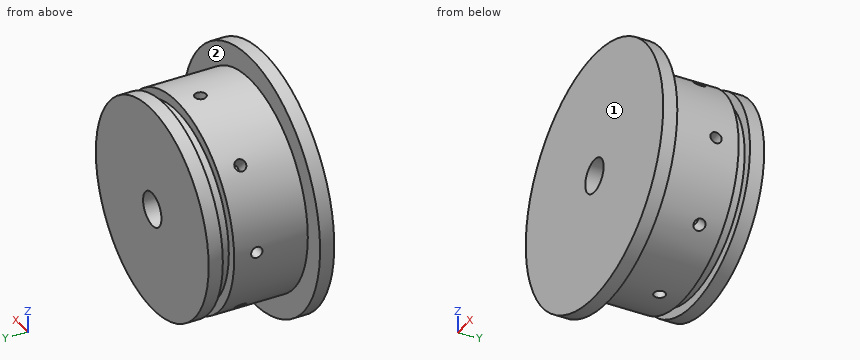
```python
from build123d import *

# Parameters (mm, degrees)
SKETCH1_R           = 45
BOSS_EXTRUDE1_DEPTH = 40
SKETCH2_R           = 45
SKETCH2_R_2         = 36.95
CUT_EXTRUDE1_DEPTH  = 35
SKETCH5_W           = 3.5
SKETCH5_H           = 4
SKETCH6_R           = 2
CUT_EXTRUDE4_DEPTH  = 46
SKETCH8_R           = 2
BOSS_EXTRUDE2_DEPTH = 30
CIRPATTERN1_COUNT   = 8
SKETCH4_R           = 6
CUT_EXTRUDE3_DEPTH  = 77


with BuildPart() as part:
    # Sketch1 → Boss-Extrude1 (new body)
    with BuildSketch(Plane(origin=(0, 0, 0), x_dir=(1, 0, 0), z_dir=(0, 1, 0))):
        Circle(SKETCH1_R)
    extrude(amount=BOSS_EXTRUDE1_DEPTH)

    # Sketch2 → Cut-Extrude1 (cut)
    with BuildSketch(Plane(origin=(0, 40, 0), x_dir=(1, 0, 0), z_dir=(0, 1, 0))):
        Circle(SKETCH2_R)
        Circle(SKETCH2_R_2, mode=Mode.SUBTRACT)
    extrude(amount=-CUT_EXTRUDE1_DEPTH, mode=Mode.SUBTRACT)

    # Sketch5 → Cut-Revolve1 (revolve, cut)
    with BuildSketch(Plane.XY):
        with Locations((-35.2, 33)):
            Rectangle(SKETCH5_W, SKETCH5_H)
    revolve(axis=Axis((0, 0, 0), (0, 1, 0)), mode=Mode.SUBTRACT)

    # Sketch6 → Cut-Extrude4 (cut)
    with BuildSketch(Plane.XY):
        with Locations((0, 23)):
            Circle(SKETCH6_R)
    cut_extrude4 = extrude(amount=-CUT_EXTRUDE4_DEPTH, mode=Mode.SUBTRACT)

    # Sketch8 → Boss-Extrude2 (add)
    with BuildSketch(Plane(origin=(0, 0, 0), x_dir=(-1, 0, 0), z_dir=(0, 0, -1))):
        with Locations((0, 23)):
            Circle(SKETCH8_R)
    boss_extrude2 = extrude(amount=BOSS_EXTRUDE2_DEPTH)

    # CirPattern1: Cut-Extrude4, Boss-Extrude2 ×8 about axis
    cirpattern1_axis = Axis((0, 0, 0), (0, 1, 0))
    for i in range(1, CIRPATTERN1_COUNT):
        add(cut_extrude4.rotate(cirpattern1_axis, i * 360 / CIRPATTERN1_COUNT), mode=Mode.SUBTRACT)
        add(boss_extrude2.rotate(cirpattern1_axis, i * 360 / CIRPATTERN1_COUNT))

    # Sketch4 → Cut-Extrude3 (cut)
    with BuildSketch(Plane.XZ):
        Circle(SKETCH4_R)
    extrude(amount=-CUT_EXTRUDE3_DEPTH, mode=Mode.SUBTRACT)


solid = part.part
```
Model file for the job. Use its own axes, mm. Face numbers are marked on the shaded views. A direction names the side the tool comes from. Coordinates: 2 decimals unless noted, no trailing zeros. Write each loop counter-clockwise with the first axis right and the second up, starting at its lowest first coordinate (ties: lowest second). Pieces come first, ordered by that corner, then holes. Notation, with made-up numbers: (84.5, 49) - (133.5, 49) arc R28 ccw to (133.5, 70) - close; hole circle Ø5 at (6.25, 36.25). An arc over 180 degrees is marked (long way). One line per question, with ' | ' between items. Start each with the question number.
Q1. Cut at D-D, the plane x = -16. List the corners of the cut face in (y, z).
Q2. Cut at A-A, the plane z = 0. List the corners of the cut face in (x, y), then the cut area to 3 significant figures.
Q3. Pin check, flat tips, straight feed: pin 1 (6 mm diameter, centred on x = 33, y = 7.5, fed in from -Z); pin 2 (1.5 mm diameter, centred on x = -18.5, y = 32.5, fed in from -Z); pin 3 (2.5 mm diameter, centred on y = 23, z = 0, fed in from -X). Stop position of each tip, or through.
Q4. 3-axis set-ups, long thin cutter, end or side, ignore diameter. For the marked faces 1 and 2: which of +Z, -Z, +X, -X, +Y, -Y reach the whole face in a straight line?
Q5. Drill centre lines: line 1 (Y direction, x = -34.5, z = 0); line 2 (Y direction, x = 32.5, z = 0); line 3 (Y direction, x = -30.5, z = 15). Where is each one in solid material? Low to high. Write a range as [from, to].
Q6. Cut at B-B, the plane x = -3.5. List the corners of the cut face in (y, z), then the cut area to 3 significant figures.
Answer below:
1) outline: (0, -42.06) - (5, -42.06) - (5, -33.31) - (31, -33.31) - (31, -29.38) - (35, -29.38) - (35, -33.31) - (40, -33.31) - (40, 33.31) - (35, 33.31) - (35, 29.38) - (31, 29.38) - (31, 33.31) - (5, 33.31) - (5, 42.06) - (0, 42.06) - close
2) outline: (-45, 0) - (-6, 0) - (-6, 40) - (-36.95, 40) - (-36.95, 35) - (-33.45, 35) - (-33.45, 31) - (-36.95, 31) - (-36.95, 25) - (-30, 25) - (-30, 21) - (-36.95, 21) - (-36.95, 5) - (-45, 5) - close; (6, 0) - (45, 0) - (45, 5) - (36.95, 5) - (36.95, 21) - (30, 21) - (30, 25) - (36.95, 25) - (36.95, 31) - (33.45, 31) - (33.45, 35) - (36.95, 35) - (36.95, 40) - (6, 40) - close | area: 2,470 mm^2
3) pin 1: z = -32.29 | pin 2: z = -28.35 | pin 3: x = -30
4) face 1: +Z, -Z, +X, -X, -Y | face 2: +Y
5) line 1: [0, 21], [25, 31], [35, 40] | line 2: [0, 21], [25, 40] | line 3: [0, 31], [35, 40]
6) outline: (0, -44.86) - (5, -44.86) - (5, -36.78) - (31, -36.78) - (31, -33.27) - (35, -33.27) - (35, -36.78) - (40, -36.78) - (40, -4.87) - (0, -4.87) - close; (0, 4.87) - (40, 4.87) - (40, 36.78) - (35, 36.78) - (35, 33.27) - (31, 33.27) - (31, 36.78) - (5, 36.78) - (5, 44.86) - (0, 44.86) - close | area: 2,610 mm^2
